Geometry: final body of the model. Coordinates: model frame, mm. A direction names the side the tool comes from. Coordinates: 2 decimals unless noted, no trailing zeros. Write each loop counter-clockwise with the first axis right and the second up, starting at its lowest first coordinate (ties: lowest second). Pieces come first, ordered by that corner, then holes. Notation, with made-up numbers: (50.25, 9) -> (79.25, 9) arc R20 cw to (79.25, 16) -> close; hole circle Ø9 at (62, 34.25). An arc over 180 degrees is marked (long way). One line per item, written item: value.
Autodesk Inventor part; units mm, degrees
ref_plane "YZ Plane" through (0, 0, 0) normal (1, 0, 0) x (0, 1, 0)
ref_plane "XZ Plane" through (0, 0, 0) normal (0, 1, 0) x (-1, 0, 0)
ref_plane "XY Plane" through (0, 0, 0) normal (0, 0, 1) x (1, 0, 0)
sketch "Sketch1" plane through (0, 0, 0) normal (0, 1, 0) x (-1, 0, 0)
  line L0 (0, 9.9) -> (0, -9.9)
  line L1 (-4.7, 9.9) -> (4.7, 9.9)
  line L2 (0, 0) -> (7.31, 0)
  line L3 (4.7, 9.9) -> (7.31, 0)
  line L4 (0, 0) -> (-7.31, 0)
  line L5 (-4.7, 9.9) -> (-7.31, 0)
  line L6 (-4.7, -9.9) -> (4.7, -9.9)
  line L7 (4.7, -9.9) -> (7.31, 0)
  line L8 (-4.7, -9.9) -> (-7.31, 0)
  line L9 (0, 9.9) -> (0, 5.69)
  line L10 (0, 5.69) -> (0.715, 5.69)
  line L11 (0.715, 5.69) -> (0.715, 4.26)
  line L12 (0.715, 4.26) -> (-0.715, 4.26)
  line L13 (-0.715, 4.26) -> (-0.715, 5.69)
  line L14 (-0.715, 5.69) -> (0, 5.69)
  circle A0 centre (0, 4.975) radius 2.2
  line L15 (0, -5.69) -> (0.715, -5.69)
  line L16 (0.715, -5.69) -> (0.715, -4.26)
  line L17 (0.715, -4.26) -> (-0.715, -4.26)
  line L18 (-0.715, -4.26) -> (-0.715, -5.69)
  line L19 (-0.715, -5.69) -> (0, -5.69)
  circle A1 centre (0, -4.975) radius 2.2
  point P0 (0, -9.9)
  dimension "d0" = 19.8
  dimension "d1" = 0
  dimension "d2" = 0
  dimension "d3" = 9.4
  dimension "d5" = 7.31
  dimension "d6" = 4.21
  dimension "d7" = 0.715
  dimension "d8" = 1.43
  dimension "d9" = 1.43
  dimension "d10" = 4.4
extrude "Extrusion1" add sketch "Sketch1" against normal blind 2.21 contours L1 L3 L2 L0 A0 | L0 A0 L4 L5 L1 | L4 L0 A1 L6 L8 | L7 L6 L0 A1 L2
extrude "Extrusion2" add sketch "Sketch1" against normal blind 2.21 contours A0 L0 L12 L11 L10 | L0 L14 L13 L12 A0 | A1 L0 L15 L16 L17 | L0 L17 L18 L19 A1
extrude "Extrusion3" add sketch "Sketch1" along normal blind 0.8 contours A0 L0 L12 L11 L10 | L0 L14 L13 L12 A0 | A1 L0 L15 L16 L17 | L0 L17 L18 L19 A1
fillet "Fillet1" radius 0.5 1 edges at (2.2, 0.8, 4.975)
fillet "Fillet2" radius 0.5 1 edges at (2.2, 0.8, -4.975)
fillet "Fillet3" radius 1.8 6 edges at (6.005, 0, -4.95) (6.005, 0, 4.95) (0, 0, -9.9) (-6.005, 0, -4.95) (-6.005, 0, 4.95) (0, 0, 9.9)
(1) First-contact query: pin 1 (1.6 mm diameter, centred on y = -0.5, z = 4.5, fed in from +X); pin 2 (1.6 mm diameter, centred on y = -1, z = -5, fed in from -X); pin 3 (1.5 mm diameter, centred on x = -3, z = -4.5, fed in from +Y). Flat tips, straight axial feed; report the tip coordinate or a pass-through.
Responses:
pin 1: stops at x = 6.12
pin 2: stops at x = -6.13
pin 3: stops at y = 0
(2) Reachability of faces 1 (the flat face through (0, 0, 0)), 2 (the cylindrical face through (-5.5, -0.51, -4.74)), 3 (the flat face through (0, -1, -4.26)) from +Z, -Z, +X, -X, +Y, -Y: full face, straight path, thin tool, end or side. Return the list, or none.
Responses:
face 1: +Y
face 2: -Z, -X, +Y
face 3: +Y, -Y
(3) Pull-direction query (X, two-part tool) for faces 4 (the flat face through (0, -1, -5.69)), 5 (the cylindrical face through (-5.527, -0.541, 4.75)), 6 (the cylindrical face through (5.527, -0.541, -4.75)); classes: released by +X, released by -X, zero draft, split by the parting line, or undercut.
Responses:
face 4: undercut
face 5: released by -X
face 6: released by +X
(4) Line query: line 1 (Z direction, x = 0, y = -0.35); line 2 (Z direction, x = -1, y = 0.15); line 3 (Y direction, x = -3.5, z = 6.25). Output: solid intervals per line, ascending. Write a range as [from, to].
Responses:
line 1: z = [-9.17, -5.69], [-4.26, 4.26], [5.69, 9.17]
line 2: z = [-6.93, -3.02], [3.02, 6.93]
line 3: y = [-2.21, 0]
(5) Section A-A (x = 0). Return the cut outline in (y, z) (3 decimals).
Responses:
outline: (-2.21, -9.9) -> (-1.8, -9.9) arc R1.8 ccw to (0, -8.1) -> (0, -7.175) -> (0.3, -7.175) arc R0.5 ccw to (0.8, -6.675) -> (0.8, -5.69) -> (-2.21, -5.69) -> close; (-2.21, -4.26) -> (0.8, -4.26) -> (0.8, -3.275) arc R0.5 ccw to (0.3, -2.775) -> (0, -2.775) -> (0, 2.775) -> (0.3, 2.775) arc R0.5 ccw to (0.8, 3.275) -> (0.8, 4.26) -> (-2.21, 4.26) -> close; (-2.21, 5.69) -> (0.8, 5.69) -> (0.8, 6.675) arc R0.5 ccw to (0.3, 7.175) -> (0, 7.175) -> (0, 8.1) arc R1.8 ccw to (-1.8, 9.9) -> (-2.21, 9.9) -> close
(6) Section B-B (y = -1.25). Return the cut outline in (x, z) (3 decimals), then the cut area to 3 significant figures.
Responses:
outline: (-7.221, 0) -> (-4.634, -9.814) -> (4.634, -9.814) -> (7.221, 0) -> (4.634, 9.814) -> (-4.634, 9.814) -> close; hole (-0.715, -5.69) -> (0.715, -5.69) -> (0.715, -4.26) -> (-0.715, -4.26) -> close; hole (-0.715, 4.26) -> (0.715, 4.26) -> (0.715, 5.69) -> (-0.715, 5.69) -> close
area: 229 mm2
